Model file for the job. Use its own axes, mm. Give positions to 0.01 mm unless a question says otherwise; leave off trailing zeros. Loops run counter-clockwise (first coordinate to the right, second up) from the corner with the lowest first, then second, coordinate; pieces in that order, holes last. Notation, with made-up numbers: (36.5, -7.75) - (58.5, -7.75) arc R21 cw to (58.5, 23.25) - close; hole circle Ø8 at (60.25, 16). An arc over 180 degrees is marked (long way). Use a Markdown table: item, result.
from build123d import *

# Parameters (mm, degrees)
PAD003_DEPTH    = 2
POCKET004_DEPTH = 22.5
POCKET005_DEPTH = 10.058462


with BuildPart() as part:
    # Sketch010 → Pad003 (new body)
    with BuildSketch(Plane.XZ):
        with BuildLine():
            Line((-4.284857, 0), (4.284857, 0))
            Line((4.284857, 0), (4.284857, 22.5))
            Line((4.284857, 22.5), (5, 84))
            ThreePointArc((5, 84), (0, 89), (-5, 84))
            Line((-4.284857, 22.5), (-5, 84))
            Line((-4.284857, 22.5), (-4.284857, 0))
        make_face()
    extrude(amount=PAD003_DEPTH)

    # Sketch011 (on Face1 of Pad003) → Pocket004 (cut)
    with BuildSketch(Plane(origin=(0, 0, 0), x_dir=(1, 0, 0), z_dir=(0, 0, -1))):
        Polygon((-3.284857, 2), (-3.284857, 1), (-8.284857, 1), (-8.284857, 5.501038), align=None)
        Polygon((8.284857, 5.501038), (3.284857, 2), (3.284857, 1), (8.284857, 1), align=None)
    extrude(amount=-POCKET004_DEPTH, mode=Mode.SUBTRACT)

    # Sketch012 (on Face12 of Pocket004) → Pocket005 (cut, through all)
    with BuildSketch(Plane(origin=(-4.022675, 0, -0.046777), x_dir=(0.011628, 0, -0.999932), z_dir=(-0.999932, 0, -0.011628))):
        Polygon((-89.452459, 0.2), (-22.548301, 2), (-89.452459, 14.03), align=None)
    extrude(amount=-POCKET005_DEPTH, mode=Mode.SUBTRACT)


with BuildPart() as part_1:
    # Body001 placement: moved
    add(part.part.moved(Location((0, 25, 0))))


solid = part_1.part
(1) Slice it at D-D, the plane z = 52. Write the cut outline in (x, y).
Computed:
| item | result |
|---|---|
| outline | (-4.63, 23.79) - (4.63, 23.79) - (4.63, 25) - (-4.63, 25) - close |
(2) Slice it at B-B, the plane y = 23.7. Write the cut outline in (x, z).
Computed:
| item | result |
|---|---|
| outline | (-4.59, 48.52) - (-4.28, 22.5) - (-3.28, 22.5) - (-3.28, 0) - (3.28, 0) - (3.28, 22.5) - (4.28, 22.5) - (4.59, 48.62) - close |
(3) Drill centre lines: probe 1 along X at (y, z) = (23.3, 13.5); probe 2 along Y at (x, z) = (-2, 54.5); probe 3 along X at (y, z) = (24.05, 39.5). Where is each one in solid material? Low to high. Write a range as [from, to].
Computed:
| item | result |
|---|---|
| probe 1 | [-3.28, 3.28] |
| probe 2 | [23.86, 25] |
| probe 3 | [-4.48, 4.48] |
(4) Slice it at C-C, the plane x = 1.75. Write the cut outline in (y, z), plus the area to 3 significant figures.
Computed:
| item | result |
|---|---|
| outline | (23, 0) - (25, 0) - (25, 88.68) - (24.78, 88.68) - (23, 22.57) - close |
| area | 119 mm² |
(5) Pin check, flat tips, straight feed: P1, Ø0.8, axis at x = 4, y = 23.5, coming from the -Z side; P2, Ø0.8, axis at x = -4, z = 14, coming from the -Y side; P3, Ø1.1, axis at y = 23.5, z = 15, coming from the -X side. Stop position of each tip, or through.
Computed:
| item | result |
|---|---|
| P1 | z = 22.5 |
| P2 | y = 24 |
| P3 | x = -4.28 |
(6) Slice it at A-A, the plane z = 9. Write the cut outline in (x, y), plus the area to 3 significant figures.
Computed:
| item | result |
|---|---|
| outline | (-4.28, 24) - (-3.28, 24) - (-3.28, 23) - (3.28, 23) - (3.28, 24) - (4.28, 24) - (4.28, 25) - (-4.28, 25) - close |
| area | 15.1 mm² |
